```python
from build123d import *

# Parameters (mm, degrees)
SKETCH1_R           = 12.7
SKETCH1_R_2         = 11.1125
SKETCH1_R_3         = 3.175
BOSS_EXTRUDE1_DEPTH = 2.54
SKETCH1_3_R         = 11.1125
SKETCH1_3_R_2       = 3.175
BOSS_EXTRUDE2_DEPTH = 47.625
CHAMFER1_SIZE       = 2.54
CHAMFER1_SIZE2      = 1.27
SKETCH2_R           = 2.286
BOSS_EXTRUDE3_DEPTH = 2.38125
FILLET1_R           = 3.175
FILLET2_R           = 3.175


with BuildPart() as part:
    # Sketch1 → Boss-Extrude1 (new body)
    # profile 1 of 3: a face of its own
    with BuildSketch(Plane.XY):
        Circle(SKETCH1_R)
        Circle(SKETCH1_R_2, mode=Mode.SUBTRACT)
    # profile 2 of 3: a face of its own
    with BuildSketch(Plane.XY):
        Circle(SKETCH1_R_2)
        Circle(SKETCH1_R_3, mode=Mode.SUBTRACT)
    # profile 3 of 3: a face of its own
    with BuildSketch(Plane.XY):
        Circle(SKETCH1_R_3)
    extrude(amount=BOSS_EXTRUDE1_DEPTH)

    # Sketch1<3> → Boss-Extrude2 (add)
    with BuildSketch(Plane.XY):
        Circle(SKETCH1_3_R)
        Circle(SKETCH1_3_R_2, mode=Mode.SUBTRACT)
    extrude(amount=BOSS_EXTRUDE2_DEPTH)

    # Chamfer1
    chamfer1_edges = [part.edges().sort_by_distance(p)[0] for p in [
        (-12.7, 0, 0),
    ]]
    chamfer1_side = [part.faces().sort_by_distance(p)[0] for p in [
        (0, 0, 0),
    ]]
    chamfer(chamfer1_edges, length=CHAMFER1_SIZE, length2=CHAMFER1_SIZE2, reference=chamfer1_side[0])

    # Sketch2 → Boss-Extrude3 (add, symmetric)
    with BuildSketch(Plane(origin=(0, 0, 0), x_dir=(1, 0, 0), z_dir=(0, 1, 0))):
        with BuildLine():
            Line((-4.240295204, 11.693248793), (-11.1125, -1.74625))
            Line((-11.1125, -1.74625), (11.1125, -1.74625))
            Line((11.1125, -1.74625), (4.240295204, 11.693248793))
            ThreePointArc((4.240295204, 11.693248793), (0, 14.2875), (-4.240295204, 11.693248793))
        make_face()
        with Locations(Location((0, 9.525, 0), (0, 0, 90))):
            Circle(SKETCH2_R, mode=Mode.SUBTRACT)
    extrude(amount=BOSS_EXTRUDE3_DEPTH, both=True)

    # Fillet1
    fillet1_edges = [part.edges().sort_by_distance(p)[0] for p in [
        (10.263836295, -1.194873852, 0.086576696),
        (-10.240026318, 0, 0.040013159),
        (10.263836295, 1.194873852, 0.086576696),
    ]]
    fillet(fillet1_edges, radius=FILLET1_R)

    # Fillet2
    fillet2_edges = [part.edges().sort_by_distance(p)[0] for p in [
        (0, 2.38125, 0),
        (0, -2.38125, 0),
    ]]
    fillet(fillet2_edges, radius=FILLET2_R)


solid = part.part
```
Can you work these out from the model? Positions are in its coordinate system, mm. A direction names the side the tool comes from. Coordinates: 2 decimals unless noted, no trailing zeros. Loops run counter-clockwise (first coordinate to the right, second up) from the corner with the lowest first, then second, coordinate; pieces in that order, holes last.
Item 1: Please list where these lines run through material, in increasing order: L1, parallel to Y at x = 0, z = 41.5 (1 decimal); L2, parallel to Z at x = 6.5, y = 6.75 (3 decimals).
Answers below:
L1: y = -11.1 to -3.2, 3.2 to 11.1
L2: z = 0 to 47.625
Item 2: Which directions (+Z, -Z, +X, -X, +Y, -Y) give clear straight access to the entire face, cutting with the end or side of a thin tool? Please do faces 4 (the face through (-2.75, -12.4, 1.9)), 5 (the face through (10.6, 3.34, 24.77)), 6 (the face through (0, -7, 0)), 7 (the face through (0, 7, 0)).
Answers below:
face 4: +Z, -Z
face 5: +Z
face 6: -Z, +X, -X, -Y
face 7: -Z, +X, -X, +Y
Item 3: I'm going to push flat-ended pins straight in: pin 1 (4 mm diameter, centred on y = -5.5, z = 5, fed in from +X); pin 2 (1.5 mm diameter, centred on x = -5.5, y = -2, fed in from -Z); pin 3 (1.5 mm diameter, centred on x = 3.5, z = 17.5, fed in from +Y). Where does each tip first touch, or does it pass through?
Answers below:
pin 1: stops at x = 10.55
pin 2: stops at z = -10.7
pin 3: stops at y = 10.77
Item 4: Suppose I cut it at B-B (z = -8). Please give me the cut outline in (x, y).
Answers below:
outline: (-6.13, -2.38) - (-1.7, -2.38) - (-1.7, 2.38) - (-6.13, 2.38) - close; (1.7, -2.38) - (6.13, -2.38) - (6.13, 2.38) - (1.7, 2.38) - close
Item 5: If we mould it in two halves opening along Z, with no side actions, what happens to faces 1 (the face through (-0.1, -0.03, -7.24)), 2 (the face through (7.1, 0, -6.1)), 3 (the face through (0.88, -11.23, 2.54))? For each: released by +Z, released by -Z, zero draft, split by the parting line, or undercut.
Answers below:
face 1: undercut
face 2: released by -Z
face 3: released by +Z
